Geometry check sheet. Reference: the model listing, model coordinates, mm. Face numbers are marked on the shaded views. A direction names the side the tool comes from. Round coordinates to 2 decimals unless told otherwise and drop trailing zeros. Use one line per item in the form item = value.
from build123d import *

# Parameters (mm, degrees)
SKETCH1_R               = 5
SKETCH1_R_2             = 2.5
BOSS_EXTRUDE1_DEPTH     = 105
FILLET1_R               = 10
CUT_EXTRUDE1_DEPTH      = 117.542660484
CUT_EXTRUDE1_DEPTH_BACK = 117.542660484


with BuildPart() as part:
    # Sketch1 → Boss-Extrude1 (new body)
    with BuildSketch(Plane(origin=(0, 0, 0), x_dir=(0, 0, -1), z_dir=(1, 0, 0))):
        with BuildLine():
            add(Edge.make_bspline(
                [(3.73e-07, 7.5), (-15, 0), (-3.73e-07, -7.5)],
                knots=[0, 0, 0, 1, 1, 1], degree=2, weights=[1, 2.333333333, 1]))
            add(Edge.make_bspline(
                [(3.73e-07, 7.5), (100, 0), (-3.73e-07, -7.5)],
                knots=[0, 0, 0, 1, 1, 1], degree=2, weights=[1, 1.001467765, 1]))
        make_face()
        Circle(SKETCH1_R, mode=Mode.SUBTRACT)
        with Locations((10, 0)):
            Circle(SKETCH1_R_2, mode=Mode.SUBTRACT)
    extrude(amount=BOSS_EXTRUDE1_DEPTH)

    # Fillet1
    fillet1_edges = [part.edges().sort_by_distance(p)[0] for p in [
        (52.5, 7.5, -3.73e-07),
        (52.5, -7.5, 3.73e-07),
    ]]
    fillet(fillet1_edges, radius=FILLET1_R)

    # Sketch2 → Cut-Extrude1 (cut, two sides)
    with BuildSketch(Plane(origin=(0, 0, 0), x_dir=(1, 0, 0), z_dir=(0, 1, 0))) as cut_extrude1_sk:
        with BuildLine():
            Line((75, 50.03666722), (30, 50.03666722))
            Line((30, 50.03666722), (30, 19.76833361))
            ThreePointArc((30, 19.76833361), (52.5, 4.634166805), (75, 19.76833361))
            Line((75, 19.76833361), (75, 50.03666722))
        make_face()
    extrude(amount=CUT_EXTRUDE1_DEPTH, mode=Mode.SUBTRACT)
    extrude(cut_extrude1_sk.sketch, amount=-CUT_EXTRUDE1_DEPTH_BACK, mode=Mode.SUBTRACT)


solid = part.part
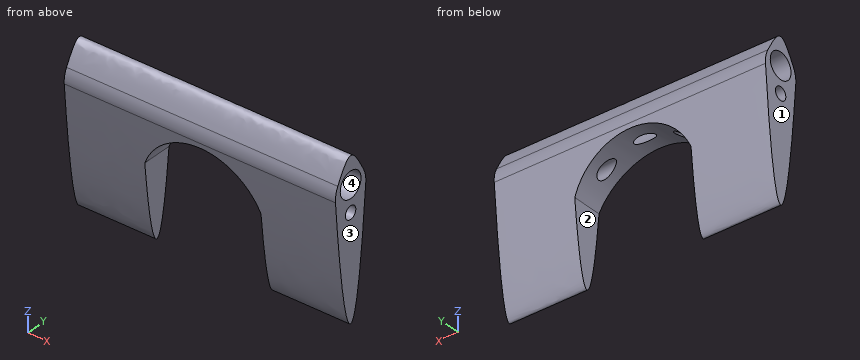
1. Mould release check, pull along Y, two halves, no side actions. Record for the marked faces 3 and 4: released by +Y, released by -Y, zero draft, split by the parting line, or undercut.
Return value:
face_3 = zero draft
face_4 = undercut
2. Tool access check on the marked faces 1 and 2. Record the directions out of +Z, -Z, +X, -X, +Y, -Y that give a thin tool (end or side, any length) a straight path to the whole face; none if there is none.
Return value:
face_1 = +Z, -Z, -X, +Y, -Y
face_2 = -Z, +Y, -Y
3. Material ranges on line 1 along X through (y, z) = (0, -28.5); line 2 along Z through (x, y) = (74, 1.75); line 3 along Z through (x, y) = (84.5, -0.25), recorded low to high.
Return value:
line_1 = 0 to 30, 75 to 105
line_2 = -17.62 to -11.79, -8.21 to -4.68, 4.68 to 9.6
line_3 = -49.98 to -12.49, -7.51 to -4.99, 4.99 to 10.48
4. Gauge pin test, flat ends, axial feed: pin 1 (4 mm diameter, centred on x = 64.5, z = 3.5, fed in from +Y); pin 2 (6 mm diameter, centred on x = 54, y = 5, fed in from -Z); pin 3 (4 mm diameter, centred on x = 16, y = -2.5, fed in from -Z). Record the tip position at first contact, or that the pin passes through.
Return value:
pin_1 = 6.67
pin_2 = -5.05
pin_3 = -49.81
5. Section check A-A (z = -10). Count the separate pieces of the cut face and the enclosed holes in it, then the cut area to 3 significant figures.
Return value:
separate_pieces = 4
enclosed_holes = 0
area = 627 mm2
